```python
from build123d import *

# Parameters (mm, degrees)
BOSS_EXTRUDE1_DEPTH = 25
SHELL1_T            = -3


with BuildPart() as part:
    # Sketch1 → Boss-Extrude1 (new body)
    with BuildSketch(Plane(origin=(0, 0, 0), x_dir=(1, 0, 0), z_dir=(0, 1, 0))):
        Polygon((-174.5, 174.5), (-174.5, -174.5), (174.5, -174.5), (174.5, 174.5), (199.5, 174.5), (199.5, -199.5), (-199.5, -199.5), (-199.5, 199.5), align=None)
    extrude(amount=BOSS_EXTRUDE1_DEPTH)

    # Shell1
    shell1_openings = [part.faces().sort_by_distance(p)[0] for p in [
        (187, 12.5, -174.5),
        (-187, 12.5, -187),
    ]]
    offset(amount=SHELL1_T, openings=shell1_openings, kind=Kind.INTERSECTION)


solid = part.part
```
Geometry check sheet. Reference: the model listing, model coordinates, mm. A direction names the side the tool comes from. Coordinates: 2 decimals unless noted, no trailing zeros. Loops run counter-clockwise (first coordinate to the right, second up) from the corner with the lowest first, then second, coordinate; pieces in that order, holes last. Notation, with made-up numbers: (-35.5, -5) - (-16.5, -5) arc R22 cw to (-16.5, 18) - close; hole circle Ø9 at (47, 51). An arc over 180 degrees is marked (long way). One line per item, written item: value. Start each with the question number.
(1) Cross-section at C-C on x = -131. Enter the section's corners in (y, z).
(2) Material ranges on line 1 (X direction, y = 8.25, z = -99.5); line 2 (Z direction, x = -59, y = 17.5); line 3 (X direction, y = 2.5, z = 123.5), recorded low to high. Write a range as [from, to].
(3) Mould release check, pull along Z, two halves, no side actions. Record for faces 1 (the flat face through (-196.5, 12, 3)), 2 (the flat face through (1, 3, 188)), 3 (the flat face through (198, 12, -174.5)): released by +Z, released by -Z, zero draft, split by the parting line, or undercut.
(4) Tool access check on faces 4 (the flat face through (-199.5, 12, 3)), 5 (the flat face through (-2, 12, 177.5)), 6 (the flat face through (177.5, 12, 4)), 7 (the flat face through (3, 12, 199.5)), 8 (the flat face through (174.5, 12, 2)). Record the directions out of +Z, -Z, +X, -X, +Y, -Y that give a thin tool (end or side, any length) a straight path to the whole face; none if there is none.
(5) Depth check by flat-ended pin: P1, Ø1.5, axis at x = -74, y = 20, coming from the -Z side; P2, Ø12.5, axis at x = 184.5, y = 6.5, coming from the -Z side. Enter the tip coordinate at first touch or a pass-through.
(6) Cross-section at A-A on z = -132.5. Enter the section's corners in (x, y), plus the area to 3 significant figures.
(7) Cross-section at B-B on y = 11.5. Enter the section's corners in (x, z).
Results below:
1. outline: (0, 174.5) - (25, 174.5) - (25, 199.5) - (0, 199.5) - close; hole (3, 177.5) - (22, 177.5) - (22, 196.5) - (3, 196.5) - close
2. line 1: x = [-199.5, -196.5], [-177.5, -174.5], [174.5, 177.5], [196.5, 199.5]
2. line 2: z = [174.5, 177.5], [196.5, 199.5]
2. line 3: x = [-199.5, -174.5], [174.5, 199.5]
3. face 1: zero draft
3. face 2: undercut
3. face 3: released by -Z
4. face 4: +Z, -Z, -X, +Y, -Y
4. face 5: none
4. face 6: -Z
4. face 7: +Z, +X, -X, +Y, -Y
4. face 8: -Z, +Y, -Y
5. P1: stops at z = 174.5
5. P2: stops at z = -174.5
6. outline: (-199.5, 0) - (-174.5, 0) - (-174.5, 25) - (-199.5, 25) - close; (174.5, 0) - (199.5, 0) - (199.5, 25) - (174.5, 25) - close; hole (-196.5, 3) - (-177.5, 3) - (-177.5, 22) - (-196.5, 22) - close; hole (177.5, 3) - (196.5, 3) - (196.5, 22) - (177.5, 22) - close
6. area: 528 mm2
7. outline: (-199.5, -199.5) - (-196.5, -196.5) - (-196.5, 196.5) - (196.5, 196.5) - (196.5, -174.5) - (199.5, -174.5) - (199.5, 199.5) - (-199.5, 199.5) - close; (-177.5, -177.5) - (-174.5, -174.5) - (-174.5, 174.5) - (174.5, 174.5) - (174.5, -174.5) - (177.5, -174.5) - (177.5, 177.5) - (-177.5, 177.5) - close
